from build123d import *

# Parameters (mm, degrees)
F_1_4_CLEARANCE_HOLE1_D = 6.5278
CIRPATTERN1_COUNT       = 6
CHAMFER1_SIZE           = 2.032
CHAMFER1_SIZE2          = 0.820981291
FILLET1_R               = 0.79375
CHAMFER2_SIZE           = 3.175


with BuildPart() as part:
    # Sketch1 → Revolve1 (revolve)
    with BuildSketch(Plane.XY, mode=Mode.PRIVATE) as revolve1_sk:
        Polygon((7.5, -69.525), (7.5, -9.006664199), (12.7, 0), (30.48, 0), (30.48, -9.525), (10.16, -9.525), (10.16, -69.525), align=None)
    revolve(revolve1_sk.sketch.rotate(Axis((0, 0, 0), (0, -1, 0)), 90), axis=Axis((0, 0, 0), (0, -1, 0)))

    # 1/4 Clearance Hole1 (through all)
    with Locations(Plane(origin=(0, 0, 0), x_dir=(1, 0, 0), z_dir=(0, 1, 0))):
        with Locations((25.4, 0)):
            f_1_4_clearance_hole1 = Hole(F_1_4_CLEARANCE_HOLE1_D / 2)

    # CirPattern1: 1/4 Clearance Hole1 ×6 about axis
    cirpattern1_axis = Axis((0, 0, 0), (0, 1, 0))
    for i in range(1, CIRPATTERN1_COUNT):
        add(f_1_4_clearance_hole1.rotate(cirpattern1_axis, i * 360 / CIRPATTERN1_COUNT), mode=Mode.SUBTRACT)

    # Chamfer1
    chamfer1_edges = [part.edges().sort_by_distance(p)[0] for p in [
        (0, -69.525, -7.5),
    ]]
    chamfer1_side = [part.faces().sort_by_distance(p)[0] for p in [
        (0, -69.525, -9.872631804),
    ]]
    chamfer(chamfer1_edges, length=CHAMFER1_SIZE, length2=CHAMFER1_SIZE2, reference=chamfer1_side[0])

    # Fillet1
    fillet1_edges = [part.edges().sort_by_distance(p)[0] for p in [
        (0, -68.704018709, -7.5),
    ]]
    fillet(fillet1_edges, radius=FILLET1_R)

    # Chamfer2
    chamfer2_edges = [part.edges().sort_by_distance(p)[0] for p in [
        (0, -9.525, -10.16),
    ]]
    chamfer(chamfer2_edges, length=CHAMFER2_SIZE)


solid = part.part
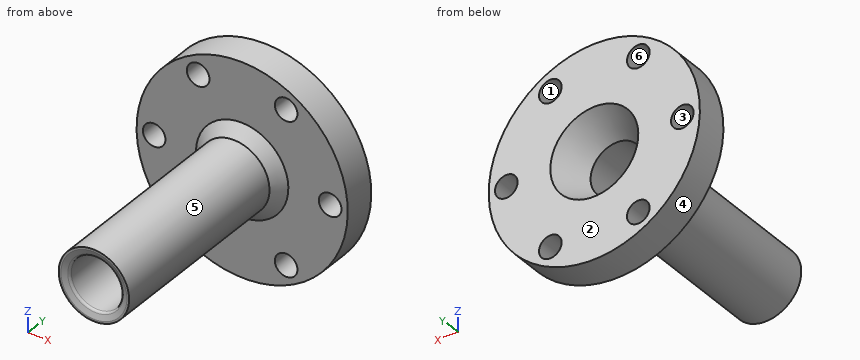
Check sheet for the modelled part. Datum: model origin and axes. Units: mm. Face numbers are marked on the shaded views. A direction names the side the tool comes from. Give positions to 0.01 mm unless a question says otherwise; leave off trailing zeros. Write each loop counter-clockwise with the first axis right and the second up, starting at its lowest first coordinate (ties: lowest second). Pieces come first, ordered by that corner, then holes. Notation, with made-up numbers: (-25, 79) -> (-5, 79) arc R25 ccw to (-5, 106) -> close; hole circle Ø11 at (59, 82.25). An arc over 180 degrees is marked (long way). One line per item, written item: value. Start each with the question number.
Item 1: Section check A-A on x = -24.5. Record the cut outline in (y, z) (3 decimals), then the cut area to 3 significant figures.
Item 2: Section check C-C on y = -21. Record the cut outline in (x, z).
Item 3: Material ranges on probe 1 along X at (y, z) = (-6.5, -23); probe 2 along Z at (x, y) = (12.7, -7); probe 3 along Y at (x, z) = (-10, 12.5) (3 decimals), recorded low to high. Write a range as from..to.
Item 4: Gauge pin test, flat ends, axial feed: pin 1 (6 mm diameter, centred on x = 10.5, y = -42.5, fed in from -Z); pin 2 (18.5 mm diameter, centred on x = -11, z = -1.5, fed in from -Y) (3 decimals); pin 3 (12 mm diameter, centred on x = -17.5, z = 3, fed in from -Y); pin 4 (8 mm diameter, centred on x = 0, y = -26.5, fed in from +Z). Record the tip position at first contact, or that the pin passes through.
Item 5: Section check B-B on z = 0. State how many separate pieces and enclosed holes the cut face has, then the cut area to 3 significant figures.
Item 6: Section check D-D on x = 25.5. Record the cut outline in (y, z) (3 decimals), then the cut area to 3 significant figures.
Item 7: Tool access check on the marked faces 5 and 6. Record the directions out of +Z, -Z, +X, -X, +Y, -Y that give a thin tool (end or side, any length) a straight path to the whole face; none if there is none.
Item 8: Draft check along Z on the marked faces 1, 2, 3 and 4. Enter one of: +Z half, -Z half, draft (parallel to the pull), parting line (faces both ways), or undercut.
Results list:
1. outline: (-9.525, -18.132) -> (0, -18.132) -> (0, -3.137) -> (-9.525, -3.137) -> close; (-9.525, 3.137) -> (0, 3.137) -> (0, 18.132) -> (-9.525, 18.132) -> close
1. area: 286 mm²
2. outline: circle Ø20.32 at (0, 0); hole circle Ø15 at (0, 0)
3. probe 1: -20..-15.81, -9.59..9.59, 15.81..20
3. probe 2: -27.71..-25.26, -18.73..18.73, 25.26..27.71
3. probe 3: -9.525..0
4. pin 1: z = -6.85
4. pin 2: y = -69.525
4. pin 3: y = -11.1
4. pin 4: z = 10.16
5. separate pieces: 4
5. enclosed holes: 0
5. area: 594 mm²
6. outline: (-9.525, -16.697) -> (0, -16.697) -> (0, -3.262) -> (-9.525, -3.262) -> close; (-9.525, 3.262) -> (0, 3.262) -> (0, 16.697) -> (-9.525, 16.697) -> close
6. area: 256 mm²
7. face 5: -Y
7. face 6: +Y, -Y
8. face 1: undercut
8. face 2: draft
8. face 3: undercut
8. face 4: parting line
